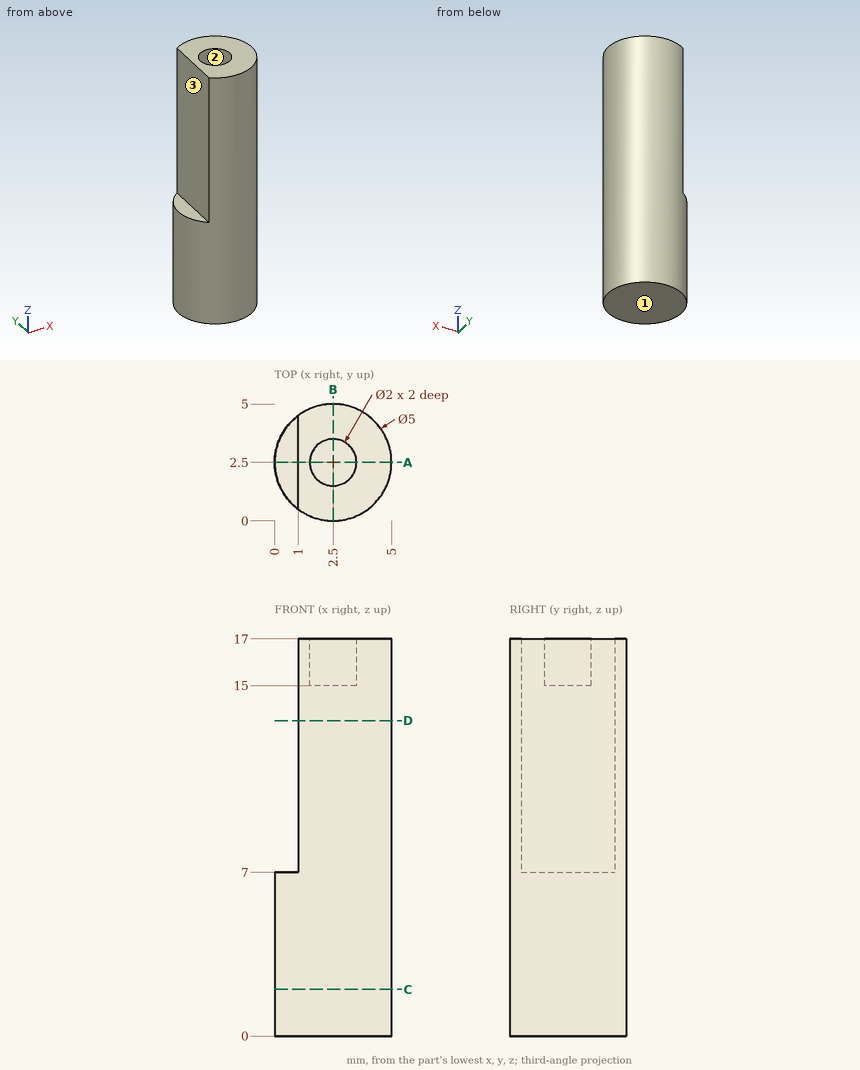
Could you check a few things on this drawing? It's one solid part, dimensions in mm from its lowest x, y, z. Round coordinates to 2 decimals unless told otherwise and drop trailing zeros. Order: outer loops, then holes, each group sorted by start corner. A loop starts at its lowest first (then second) coordinate and runs counter-clockwise, first axis right, second up.
Q1. Thinking about a two-plate mould opening in X: for the marked faces 1, 2 and 3, which applies, released by +X, released by -X, zero draft, split by the parting line, or undercut?
Geometry says:
face 1: zero draft
face 2: undercut
face 3: released by -X
Q2. Imagine slicing it at D-D, the plane z = 13.5. List the corners of the cut face in (x, y) for me.
Geometry says:
outline: (1, 0.5) arc R2.5 ccw (long way) to (1, 4.5) - close
Q3. Please list where these lines run through material, in increasing order: probe 1 along Y at (x, z) = (2.5, 16.6); probe 2 along Z at (x, y) = (3.35, 2.65); probe 3 along X at (y, z) = (2.45, 7.25).
Geometry says:
probe 1: y = 0 to 1.5, 3.5 to 5
probe 2: z = 0 to 15
probe 3: x = 1 to 5
Q4. I'm going to push flat-ended pins straight in: P1, Ø2, axis at x = 4, z = 13, coming from the -Y side; P2, Ø1.6, axis at x = 2, y = 3, coming from the +Z side. Where does each tip first touch, or does it pass through?
Geometry says:
P1: stops at y = 0.05
P2: stops at z = 17
Q5. Imagine slicing it at A-A, the plane y = 2.5. List the corners of the cut face in (x, z) for me.
Geometry says:
outline: (0, 0) - (5, 0) - (5, 17) - (3.5, 17) - (3.5, 15) - (1.5, 15) - (1.5, 17) - (1, 17) - (1, 7) - (0, 7) - close
Q6. Imagine slicing it at B-B, the plane x = 2.5. List the corners of the cut face in (y, z) for me.
Geometry says:
outline: (0, 0) - (5, 0) - (5, 17) - (3.5, 17) - (3.5, 15) - (1.5, 15) - (1.5, 17) - (0, 17) - close
Q7. Imagine slicing it at C-C, the plane z = 2. List the corners of the cut face in (x, y) for me.
Geometry says:
outline: circle Ø5 at (2.5, 2.5)
